```python
from build123d import *

# Parameters (mm, degrees)
BOSS_EXTRU_1_DEPTH      = 4
BOSS_EXTRU_3_DEPTH      = 50
ENL_V_MAT_EXTRU_1_DEPTH = 50
ENL_V_MAT_EXTRU_2_DEPTH = 50


with BuildPart() as part:
    # Esquisse1 → Boss.-Extru.1 (new body)
    with BuildSketch(Plane.XY):
        with BuildLine():
            Line((-11.273273273, 8.708708709), (34.726726727, 8.708708709))
            ThreePointArc((34.726726727, 8.708708709), (36.140940289, 8.122922271), (36.726726727, 6.708708709))
            Line((36.726726727, 6.708708709), (36.726726727, -9.291291291))
            ThreePointArc((36.726726727, -9.291291291), (36.140940289, -10.705504854), (34.726726727, -11.291291291))
            Line((34.726726727, -11.291291291), (-11.273273273, -11.291291291))
            ThreePointArc((-11.273273273, -11.291291291), (-12.687486836, -10.705504854), (-13.273273273, -9.291291291))
            Line((-13.273273273, -9.291291291), (-13.273273273, 6.708708709))
            ThreePointArc((-13.273273273, 6.708708709), (-12.687486836, 8.122922271), (-11.273273273, 8.708708709))
        make_face()
    extrude(amount=BOSS_EXTRU_1_DEPTH)

    # Esquisse2 → Boss.-Extru.3 (add)
    with BuildSketch(Plane.XY.offset(4)):
        with BuildLine():
            Line((31.726726727, 8.708708709), (34.726726727, 8.708708709))
            ThreePointArc((34.726726727, 8.708708709), (36.140940289, 8.122922271), (36.726726727, 6.708708709))
            Line((36.726726727, 6.708708709), (36.726726727, -9.291291291))
            ThreePointArc((36.726726727, -9.291291291), (36.140940289, -10.705504854), (34.726726727, -11.291291291))
            Line((34.726726727, -11.291291291), (31.726726727, -11.291291291))
            Line((31.726726727, -11.291291291), (31.726726727, 8.708708709))
        make_face()
    extrude(amount=BOSS_EXTRU_3_DEPTH)

    # Esquisse3 → Enlèv. mat.-Extru.1 (cut)
    with BuildSketch(Plane.XY.offset(4)):
        with BuildLine():
            Line((-4.273273273, 1.708708709), (11.726726727, 1.708708709))
            ThreePointArc((11.726726727, 1.708708709), (12.433833508, 1.41581549), (12.726726727, 0.708708709))
            Line((12.726726727, 0.708708709), (12.726726727, -3.291291291))
            ThreePointArc((12.726726727, -3.291291291), (12.433833508, -3.998398072), (11.726726727, -4.291291291))
            Line((11.726726727, -4.291291291), (-4.273273273, -4.291291291))
            ThreePointArc((-4.273273273, -4.291291291), (-4.980380054, -3.998398072), (-5.273273273, -3.291291291))
            Line((-5.273273273, -3.291291291), (-5.273273273, 0.708708709))
            ThreePointArc((-5.273273273, 0.708708709), (-4.980380054, 1.41581549), (-4.273273273, 1.708708709))
        make_face()
    extrude(amount=-ENL_V_MAT_EXTRU_1_DEPTH, mode=Mode.SUBTRACT)

    # Esquisse4 → Enlèv. mat.-Extru.2 (cut)
    with BuildSketch(Plane.ZY.offset(-31.726726727)):
        with BuildLine():
            Line((29, 1.708708709), (45, 1.708708709))
            ThreePointArc((45, 1.708708709), (45.707106781, 1.41581549), (46, 0.708708709))
            Line((46, 0.708708709), (46, -3.291291291))
            ThreePointArc((46, -3.291291291), (45.707106781, -3.998398072), (45, -4.291291291))
            Line((45, -4.291291291), (29, -4.291291291))
            ThreePointArc((29, -4.291291291), (28.292893219, -3.998398072), (28, -3.291291291))
            Line((28, -3.291291291), (28, 0.708708709))
            ThreePointArc((28, 0.708708709), (28.292893219, 1.41581549), (29, 1.708708709))
        make_face()
    extrude(amount=-ENL_V_MAT_EXTRU_2_DEPTH, mode=Mode.SUBTRACT)


solid = part.part
```
Read the model definition and answer for the solid it produces. Units are mm, in the model's axes. A direction names the side the tool comes from. Coordinates: 2 decimals unless noted, no trailing zeros. Write each loop counter-clockwise with the first axis right and the second up, starting at its lowest first coordinate (ties: lowest second). Pieces come first, ordered by that corner, then holes. Notation, with made-up numbers: (-10, 44) -> (0, 44) arc R30 cw to (0, 76) -> close; hole circle Ø5 at (47.25, -7). An arc over 180 degrees is marked (long way). Answer as a JSON object with one key per item and string values.
Q1. A tool of negligible diameter and unlimited length cuts with its end or side. For faces 1 (the flat face through (31.727, -1, 23)), 2 (the flat face through (-5.273, -1, 2)), 3 (the flat face through (34, -4.291, 37)), from which of +Z, -Z, +X, -X, +Y, -Y can it reach the whole face along a straight path? Write none if from no direction.
The answers:
{"face 1": "+Z, -X, +Y, -Y", "face 2": "+Z, -Z", "face 3": "+X, -X"}
Q2. The part is cut by section D-D on y = 6. Give the vertices of the cut face in (x, z).
The answers:
{"outline": "(-13.27, 0) -> (36.73, 0) -> (36.73, 54) -> (31.73, 54) -> (31.73, 4) -> (-13.27, 4) -> close"}
Q3. Determine the mould class of faces 4 (the cylindrical face through (36.156, -10.69, 26.622)), 5 (the flat face through (34, -1, 46)), 6 (the flat face through (36.727, -1, 27)) for opening direction Y: pulls with the +Y half, pulls with the -Y half, needs draft (parallel to the pull), parting line crosses it, or undercut.
The answers:
{"face 4": "pulls with the -Y half", "face 5": "undercut", "face 6": "needs draft"}
Q4. The part is cut by section B-B on z = 33.5. Give the vertices of the cut face in (x, y), then the cut area to 3 significant figures.
The answers:
{"outline": "(31.73, -11.29) -> (34.73, -11.29) arc R2 ccw to (36.73, -9.29) -> (36.73, -4.29) -> (31.73, -4.29) -> close; (31.73, 1.71) -> (36.73, 1.71) -> (36.73, 6.71) arc R2 ccw to (34.73, 8.71) -> (31.73, 8.71) -> close", "area": "68.3 mm2"}
Q5. The part is cut by section A-A on y = -0.75. Give the vertices of the cut face in (x, z).
The answers:
{"outline": "(-13.27, 0) -> (-5.27, 0) -> (-5.27, 4) -> (-13.27, 4) -> close; (12.73, 0) -> (36.73, 0) -> (36.73, 28) -> (31.73, 28) -> (31.73, 4) -> (12.73, 4) -> close; (31.73, 46) -> (36.73, 46) -> (36.73, 54) -> (31.73, 54) -> close"}
Q6. Flat-ended cylindrical pins translate along their axes: pin 1 Ø12 at (y, z) = (-8.5, 13) entering from -X; pin 2 Ø1.5 at (y, z) = (-3, 36) entering from +X; pin 3 Ø10 at (x, y) = (10.5, -4.5) entering from +Z. Find the tip coordinate at first contact, or state that the pin passes through.
The answers:
{"pin 1": "stops at x = 31.73", "pin 2": "passes through", "pin 3": "stops at z = 4"}
Q7. The part is cut by section C-C on x = 6.5. Give the vertices of the cut face in (y, z).
The answers:
{"outline": "(-11.29, 0) -> (-4.29, 0) -> (-4.29, 4) -> (-11.29, 4) -> close; (1.71, 0) -> (8.71, 0) -> (8.71, 4) -> (1.71, 4) -> close"}
Q8. Consider line 1 (X direction, y = -4.75, z = 41); line 2 (Z direction, x = 33.5, y = -1.75); line 3 (Z direction, x = -11, y = -1.25). Determine where each line is inside the solid, lowest interval first. Write a range as [from, to].
The answers:
{"line 1": "x = [31.73, 36.73]", "line 2": "z = [0, 28], [46, 54]", "line 3": "z = [0, 4]"}
